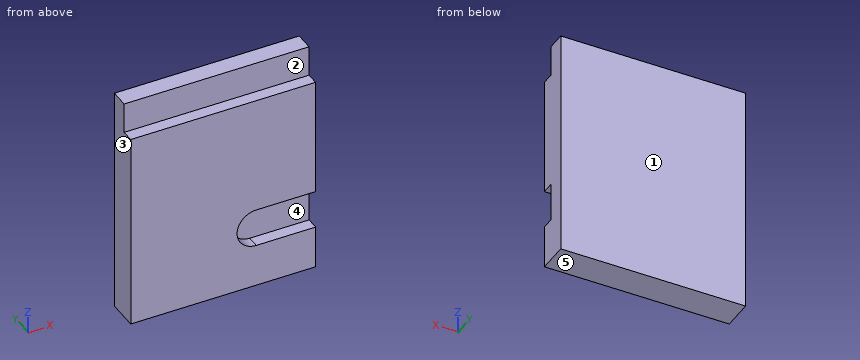
from build123d import *

# Parameters (mm, degrees)
F0_W     = 120
F0_H     = 20
F1_DEPTH = 12
F2_DEPTH = 20
F3_DEPTH = 20
F4_DEPTH = 20
F5_DEPTH = 12


with BuildPart() as f1:
    # F0 (on Front) → F1 (new body)
    with BuildSketch(Plane.XZ):
        with Locations((-60, 55.987342)):
            Rectangle(F0_W, F0_H)
    extrude(amount=F1_DEPTH)

    # F0 (on Front) → F2 (join)
    with BuildSketch(Plane.XZ):
        Polygon((0, 45.987342), (-120, 45.987342), (-120, -31.012658), (-38.5, -31.012658), (0, -31.012658), align=None)
    extrude(amount=F2_DEPTH)

    # F0 (on Front) → F3 (join)
    with BuildSketch(Plane.XZ):
        with BuildLine():
            Line((-38.5, -31.012658), (-120, -31.012658))
            Line((-120, -31.012658), (-120, -56.012658))
            Line((-120, -56.012658), (-38.5, -56.012658))
            ThreePointArc((-38.5, -56.012658), (-51, -43.512658), (-38.5, -31.012658))
        make_face()
    extrude(amount=F3_DEPTH)

    # F0 (on Front) → F4 (join)
    with BuildSketch(Plane.XZ):
        Polygon((-38.5, -56.012658), (-120, -56.012658), (-120, -84.012658), (0, -84.012658), (0, -56.012658), align=None)
    extrude(amount=F4_DEPTH)

    # F0 (on Front) → F5 (join)
    with BuildSketch(Plane.XZ):
        with BuildLine():
            Line((0, -31.012658), (-38.5, -31.012658))
            ThreePointArc((-38.5, -31.012658), (-51, -43.512658), (-38.5, -56.012658))
            Line((-38.5, -56.012658), (0, -56.012658))
            Line((0, -56.012658), (0, -31.012658))
        make_face()
    extrude(amount=F5_DEPTH)


solid = f1.part
Model file for the job. Use its own axes, mm. Face numbers are marked on the shaded views. A direction names the side the tool comes from. Round coordinates to 2 decimals unless told otherwise and drop trailing zeros. Loops run counter-clockwise (first coordinate to the right, second up) from the corner with the lowest first, then second, coordinate; pieces in that order, holes last. Notation, with made-up numbers: (57, -30.5) - (90, -30.5) arc R24 cw to (90, -19.5) - close; hole circle Ø11 at (61.5, -5.75). An arc over 180 degrees is marked (long way). Write each question's results on one line, items separated by ' | '.
(1) Pin check, flat tips, straight feed: pin 1 (10 mm diameter, centred on x = -30, z = 54, fed in from -Y); pin 2 (2.5 mm diameter, centred on x = -25.5, y = -17, fed in from +Z). Stop position of each tip, or through.
Answer below:
pin 1: stops at y = -12 | pin 2: stops at z = 45.99
(2) Saw through at A-A, the plane x = -59.5. List the corners of the cut face in (y, z), then the cut area to 3 significant figures.
Answer below:
outline: (-20, -84.01) - (0, -84.01) - (0, 65.99) - (-12, 65.99) - (-12, 45.99) - (-20, 45.99) - close | area: 2,840 mm^2
(3) Wall check: L1, parallel to Z at x = -11, y = -16.75; L2, parallel to Z at x = -77.5, y = -17.25; L3, parallel to Z at x = -47.5, y = -18.5. Give the ranges that are in metal, low to high.
Answer below:
L1: z = -84.01 to -56.01, -31.01 to 45.99 | L2: z = -84.01 to 45.99 | L3: z = -84.01 to -52.19, -34.84 to 45.99
(4) Mould opens along Z. For the marked faces 3, 4 and 5 say: released by +Z, released by -Z, zero draft, split by the parting line, or undercut.
Answer below:
face 3: zero draft | face 4: undercut | face 5: released by -Z
(5) 3-axis set-ups, long thin cutter, end or side, ignore diameter. For the marked faces 1 and 2: which of +Z, -Z, +X, -X, +Y, -Y reach the whole face in a straight line?
Answer below:
face 1: +Z, -Z, +X, -X, +Y | face 2: +Z, +X, -X, -Y
(6) Saw through at B-B, the plane z = 51. List the corners of the cut face in (x, y), then the cut area to 3 significant figures.
Answer below:
outline: (-120, -12) - (0, -12) - (0, 0) - (-120, 0) - close | area: 1,440 mm^2
